Verification items for this drawing (mm, ordinates from the low corner). A direction names the side the tool comes from. Round coordinates to 2 decimals unless told otherwise and drop trailing zeros. Loops run counter-clockwise (first coordinate to the right, second up) from the corner with the lowest first, then second, coordinate; pieces in that order, holes last. Notation, with made-up numbers: M -20,-30.75 L 2,-30.75 A17 cw 2,-24.75 Z; hole C 66.5,55.5 d10. An arc over 180 degrees is marked long. One line per item, written item: value.
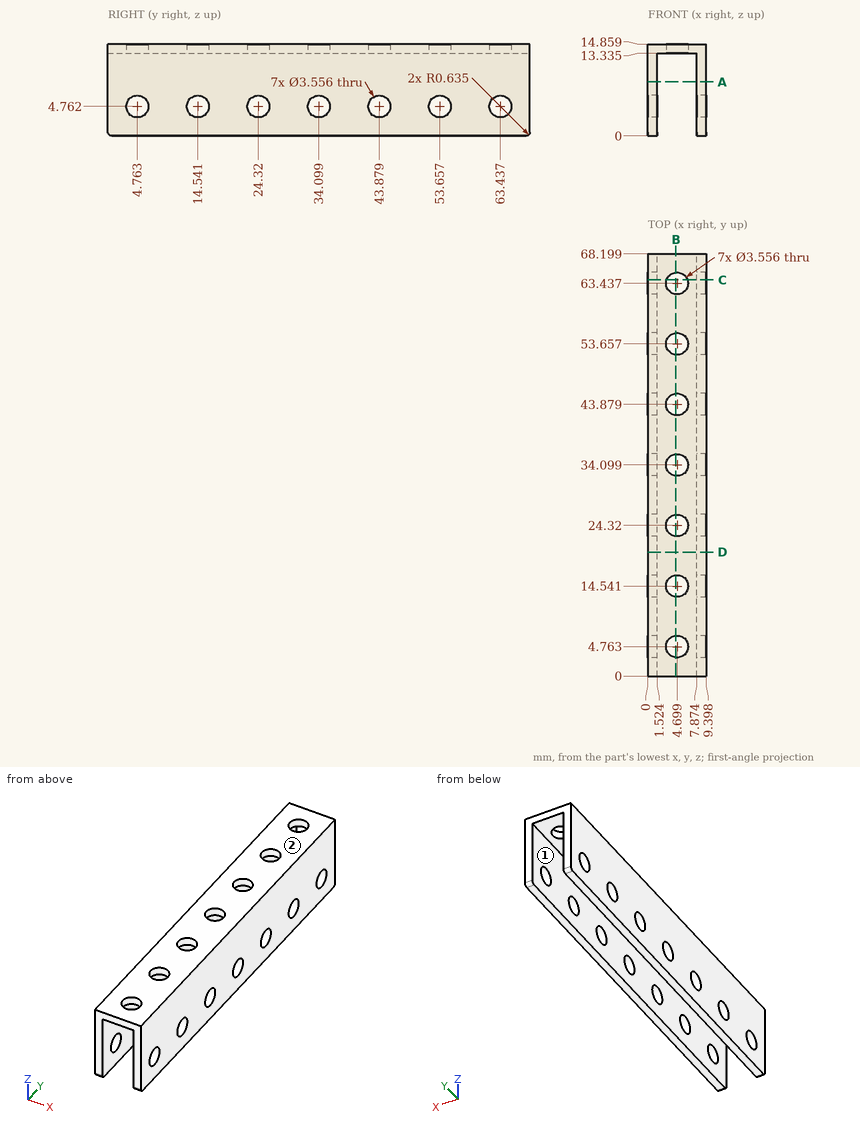
(1) Sectioned sample at D-D on y = 20. Enter the section's corners in (x, z) (1 decimal).
Completed:
outline: M 0,0 L 1.5,0 L 1.5,13.3 L 7.9,13.3 L 7.9,0 L 9.4,0 L 9.4,14.9 L 0,14.9 Z
(2) Sectioned sample at B-B on x = 4.5. Count the separate pieces of the cut face and the enclosed holes in it.
Completed:
separate pieces: 8
enclosed holes: 0
(3) Thickness scan on L1, parallel to X at y = 16, z = 11.5 (1 decimal); L2, parallel to Z at x = 9, y = 14.5 (1 decimal); L3, parallel to Z at x = 6.75, y = 49.5 (1 decimal). Record the ranges inside material, lowest first. Write a range as from..to.
Completed:
L1: x = 0..1.5, 7.9..9.4
L2: z = 0..3, 6.5..14.9
L3: z = 13.3..14.9
(4) Tool access check on the marked faces 1 and 2. Record the directions out of +Z, -Z, +X, -X, +Y, -Y that give a thin tool (end or side, any length) a straight path to the whole face; none if there is none.
Completed:
face 1: -Z, +Y, -Y
face 2: +Z, +X, -X, +Y, -Y
(5) Depth check by flat-ended pin: pin 1 Ø4.5 at (x, y) = (4.7, 4.76) entering from -Z (1 decimal); pin 2 Ø2 at (x, y) = (4.7, 53.66) entering from +Z. Enter the tip coordinate at first touch or a pass-through.
Completed:
pin 1: stops at z = 13.3
pin 2: passes through
(6) Sectioned sample at A-A on z = 8.75. Enter the section's corners in (x, y) (1 decimal).
Completed:
outline: M 0,0 L 1.5,0 L 1.5,68.2 L 0,68.2 Z; M 7.9,0 L 9.4,0 L 9.4,68.2 L 7.9,68.2 Z
(7) Sectioned sample at C-C on y = 64. Enter the section's corners in (x, z) (1 decimal).
Completed:
outline: M 0,0 L 1.5,0 L 1.5,3.1 L 0,3.1 Z; M 0,6.4 L 1.5,6.4 L 1.5,13.3 L 3,13.3 L 3,14.9 L 0,14.9 Z; M 6.4,13.3 L 7.9,13.3 L 7.9,6.4 L 9.4,6.4 L 9.4,14.9 L 6.4,14.9 Z; M 7.9,0 L 9.4,0 L 9.4,3.1 L 7.9,3.1 Z
